from build123d import *

# Parameters (mm, degrees)
SKETCH2_R                        = 1.375
BOSS_EXTRUDE1_DEPTH              = 1.75
CUT_EXTRUDE1_DEPTH               = 10
CHAMFER1_SIZE                    = 1.25
CHAMFER1_SIZE2                   = 3.434346774
CHAMFER1_EDGE_2_SIZE             = 1.25
CHAMFER1_EDGE_2_SIZE2            = 2.552275757
CHAMFER1_EDGE_3_SIZE             = 1.25
CHAMFER1_EDGE_3_SIZE2            = 2.552275757
CHAMFER1_OF_MIRROR1_SIZE2        = 3.434346774
CHAMFER1_OF_MIRROR1_SIZE         = 1.25
CHAMFER1_EDGE_2_OF_MIRROR1_SIZE2 = 2.552275757
CHAMFER1_EDGE_2_OF_MIRROR1_SIZE  = 1.25
CHAMFER1_EDGE_3_OF_MIRROR1_SIZE2 = 2.552275757
CHAMFER1_EDGE_3_OF_MIRROR1_SIZE  = 1.25
BOSS_EXTRUDE2_DEPTH              = 1
SKETCH8_R                        = 1.375
CUT_EXTRUDE2_DEPTH               = 102.267307157


with BuildPart() as part:
    # Sketch2 → Boss-Extrude1 (new body)
    with BuildSketch(Plane(origin=(0, 0, 0), x_dir=(1, 0, 0), z_dir=(0, 1, 0))):
        with BuildLine():
            Line((0, 4), (30.5, 4))
            ThreePointArc((30.5, 4), (34.5, 0), (30.5, -4))
            Line((30.5, -4), (0, -4))
            ThreePointArc((0, -4), (-4, 0), (0, 4))
        make_face()
        with Locations(Location((0, 0, 0), (0, 0, 270))):
            Circle(SKETCH2_R, mode=Mode.SUBTRACT)
        with Locations(Location((30.5, 0, 0), (0, 0, 270))):
            Circle(SKETCH2_R, mode=Mode.SUBTRACT)
    extrude(amount=BOSS_EXTRUDE1_DEPTH)

    # Sketch3 → Cut-Extrude1 (cut)
    with BuildSketch(Plane(origin=(0, 1.75, 0), x_dir=(1, 0, 0), z_dir=(0, 1, 0))):
        with BuildLine():
            Line((30.5, 4), (0, 4))
            add(Edge.make_bspline(
                [(0, 4), (1.392554105, 4), (4.712816119, 2.730302251), (11.200086309, 0.212313893), (19.274696625, 0.212313893), (25.842577961, 2.730302251), (29.028765437, 4), (30.5, 4)],
                knots=[0, 0, 0, 0, 0.131328662, 0.332777634, 0.667222366, 0.868671338, 1, 1, 1, 1], degree=3))
        make_face()
    extrude(amount=-CUT_EXTRUDE1_DEPTH, mode=Mode.SUBTRACT)

    # Sketch4 → Loft1 section 0
    with BuildSketch(Plane(origin=(0, 1.75, 0), x_dir=(1, 0, 0), z_dir=(0, 1, 0))):
        with BuildLine():
            Line((8.453738644, -1.875), (7.226869322, 0.25))
            Line((7.226869322, 0.25), (4.773130678, 0.25))
            Line((4.773130678, 0.25), (3.546261356, -1.875))
            Line((3.546261356, -1.875), (4.773130678, -4))
            Line((4.773130678, -4), (7.226869322, -4))
            Line((7.226869322, -4), (8.453738644, -1.875))
        make_face()
    # Sketch5 → Loft1 section 1
    with BuildSketch(Plane(origin=(0, 91.75, 0), x_dir=(1, 0, 0), z_dir=(0, 1, 0))):
        with BuildLine():
            Line((-5.046261356, -1.875), (-6.273130678, 0.25))
            Line((-6.273130678, 0.25), (-8.726869322, 0.25))
            Line((-8.726869322, 0.25), (-9.953738644, -1.875))
            Line((-9.953738644, -1.875), (-8.726869322, -4))
            Line((-8.726869322, -4), (-6.273130678, -4))
            Line((-6.273130678, -4), (-5.046261356, -1.875))
        make_face()
    loft1 = loft()

    # Chamfer1
    chamfer1_edges = [part.edges().sort_by_distance(p)[0] for p in [
        (6, 1.75, -0.25),
    ]]
    chamfer1_side = [part.faces().sort_by_distance(p)[0] for p in [
        (15.962582186, 1.75, 0.665337448),
    ]]
    chamfer(chamfer1_edges, length=CHAMFER1_SIZE, length2=CHAMFER1_SIZE2, reference=chamfer1_side[0])

    # Chamfer1 edge 2
    chamfer1_edge_2_edges = [part.edges().sort_by_distance(p)[0] for p in [
        (4.159696017, 1.75, 0.8125),
    ]]
    chamfer1_edge_2_side = [part.faces().sort_by_distance(p)[0] for p in [
        (15.962582186, 1.75, 0.665337448),
    ]]
    chamfer(chamfer1_edge_2_edges, length=CHAMFER1_EDGE_2_SIZE, length2=CHAMFER1_EDGE_2_SIZE2, reference=chamfer1_edge_2_side[0])

    # Chamfer1 edge 3
    chamfer1_edge_3_edges = [part.edges().sort_by_distance(p)[0] for p in [
        (4.159696017, 1.75, 2.9375),
    ]]
    chamfer1_edge_3_side = [part.faces().sort_by_distance(p)[0] for p in [
        (15.962582186, 1.75, 0.665337448),
    ]]
    chamfer(chamfer1_edge_3_edges, length=CHAMFER1_EDGE_3_SIZE, length2=CHAMFER1_EDGE_3_SIZE2, reference=chamfer1_edge_3_side[0])

    # Mirror1: Loft1 across plane
    add(loft1.mirror(Plane(origin=(15.25, 0, 0), x_dir=(0, 0, 1), z_dir=(1, 0, 0))))

    # Chamfer1 of Mirror1
    chamfer1_of_mirror1_edges = [part.edges().sort_by_distance(p)[0] for p in [
        (24.5, 1.75, -0.25),
    ]]
    chamfer(chamfer1_of_mirror1_edges, length=CHAMFER1_OF_MIRROR1_SIZE, length2=CHAMFER1_OF_MIRROR1_SIZE2)

    # Chamfer1 edge 2 of Mirror1
    chamfer1_edge_2_of_mirror1_edges = [part.edges().sort_by_distance(p)[0] for p in [
        (26.340303983, 1.75, 0.8125),
    ]]
    chamfer(chamfer1_edge_2_of_mirror1_edges, length=CHAMFER1_EDGE_2_OF_MIRROR1_SIZE, length2=CHAMFER1_EDGE_2_OF_MIRROR1_SIZE2)

    # Chamfer1 edge 3 of Mirror1
    chamfer1_edge_3_of_mirror1_edges = [part.edges().sort_by_distance(p)[0] for p in [
        (26.340303983, 1.75, 2.9375),
    ]]
    chamfer(chamfer1_edge_3_of_mirror1_edges, length=CHAMFER1_EDGE_3_OF_MIRROR1_SIZE, length2=CHAMFER1_EDGE_3_OF_MIRROR1_SIZE2)

    # Sketch6 → Boss-Extrude2 (add)
    with BuildSketch(Plane.XZ):
        with BuildLine():
            Line((9.25, 4), (9.25, -1.186704991))
            add(Edge.make_bspline(
                [(9.25, -1.186704991), (9.498756449, -1.120525729), (13.135912237, -0.212313893), (17.336765902, -0.212313893), (21.001177664, -1.119553839), (21.25, -1.185159308)],
                knots=[0.308100917, 0.308100917, 0.308100917, 0.308100917, 0.332777634, 0.667222366, 0.691706881, 0.691706881, 0.691706881, 0.691706881], degree=3))
            Line((21.25, -1.185159308), (21.25, 4))
            Line((21.25, 4), (9.25, 4))
        make_face()
    extrude(amount=BOSS_EXTRUDE2_DEPTH)

    # Sketch8 → Cut-Extrude2 (cut, through all)
    with BuildSketch(Plane.XZ.offset(1)):
        with Locations(Location((11.249999996, 1.406776311, 0), (0, 0, 270))):
            Circle(SKETCH8_R)
        with Locations(Location((19.250000004, 1.407291539, 0), (0, 0, 270))):
            Circle(SKETCH8_R)
    extrude(amount=-CUT_EXTRUDE2_DEPTH, mode=Mode.SUBTRACT)


solid = part.part
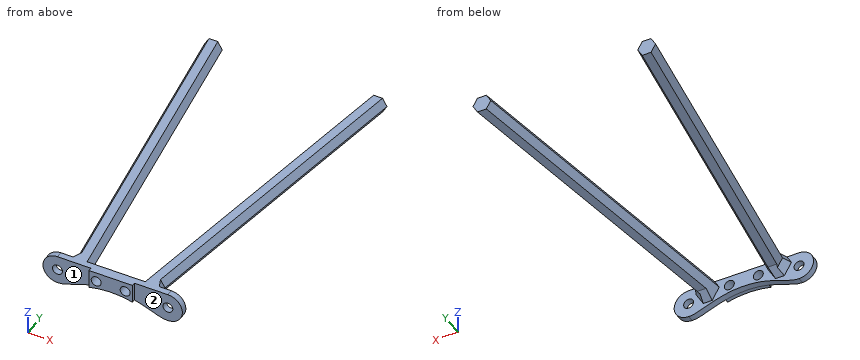
Could you check a few things on this model? Use its own coordinates, in mm. Face numbers are marked on the shaded views. A direction names the side the tool comes from. Give positions to 0.01 mm unless a question says otherwise; leave off trailing zeros. Return JSON: item names as keys, results as strings. Group by question number.
Q1. Which directions (+Z, -Z, +X, -X, +Y, -Y) give clear straight access to the entire face, cutting with the end or side of a thin tool? Please do the marked faces 1 and 2.
Q2. Will these pins go through, and if not, where does the flat tip stop? pin 1 Ø3 at (x, z) = (-3, 1) entering from -Y; pin 2 Ø1.1 at (y, z) = (-0.5, 0.5) entering from -X; pin 3 Ø3.5 at (x, z) = (11.25, 1.41) entering from -Y; pin 4 Ø0.8 at (y, z) = (-0.5, 1.5) entering from +X.
Q3. Please list where these lines run through material, in increasing order: line 1 along X through (y, z) = (0.8, 0) (3 decimals); line 2 along Z through (x, y) = (-6, 85); line 3 along X through (y, z) = (69.5, 1.25). Write a range as [from, to].
Resolved:
{
 "1": {"face 1": "+Z, -Z, -X, -Y", "face 2": "+Z, -Z, +X, -Y"},
 "2": {"pin 1": "stops at y = 0", "pin 2": "stops at x = -3.99", "pin 3": "stops at y = -1", "pin 4": "stops at x = 21.25"},
 "3": {"line 1": "x = [-4, -1.375], [1.375, 29.125], [31.875, 34.5]", "line 2": "z = [-0.25, 4]", "line 3": "x = [-6.26, -2.07], [32.57, 36.76]"}
}
